```python
from build123d import *

# Parameters (mm, degrees)
F1_DEPTH = 6.35
F2_D     = 4.7625
F3_D     = 3.571875
F4_R     = 5.08


with BuildPart() as f1:
    # F0 (on Front) → F1 (new body)
    with BuildSketch(Plane.XZ):
        Polygon((62.865, 15.748), (12.065, 25.908), (-12.065, 25.908), (-62.865, 15.748), (-62.865, -15.748), (-12.065, -25.908), (12.065, -25.908), (62.865, -15.748), align=None)
    extrude(amount=F1_DEPTH)

    # F2 (through all)
    with Locations(Plane(origin=(0, 0, 0), x_dir=(1, 0, 0), z_dir=(0, 1, 0))):
        with Locations((-13.335, -15.748), (13.335, -15.748), (13.335, 15.748), (-13.335, 15.748)):
            Hole(F2_D / 2)

    # F3 (through all)
    with Locations(Plane(origin=(0, 0, 0), x_dir=(1, 0, 0), z_dir=(0, 1, 0))):
        with Locations((26.035, -9.144), (50.165, -9.144), (50.165, 9.144), (26.035, 9.144), (-26.035, 9.144), (-26.035, -9.144), (-50.165, -9.144), (-50.165, 9.144)):
            Hole(F3_D / 2)

    # F4
    f4_edges = [f1.edges().sort_by_distance(p)[0] for p in [
        (-62.865, -3.175, 15.748),
        (62.865, -3.175, -15.748),
        (-62.865, -3.175, -15.748),
        (62.865, -3.175, 15.748),
        (12.065, -3.175, -25.908),
        (12.065, -3.175, 25.908),
        (-12.065, -3.175, -25.908),
        (-12.065, -3.175, 25.908),
    ]]
    fillet(f4_edges, radius=F4_R)


solid = f1.part
```
Input: part model. Units: mm. Frame: model coordinates. Coordinates: 2 decimals unless noted, no trailing zeros. Loops run counter-clockwise (first coordinate to the right, second up) from the corner with the lowest first, then second, coordinate; pieces in that order, holes last. Notation, with made-up numbers: (78.5, -9.75) -> (91.5, -9.75) arc R17 cw to (91.5, 18.25) -> close; hole circle Ø5 at (-40, 78). An arc over 180 degrees is marked (long way). Use a Markdown table: item, result.
1) Pull-direction query (X, two-part tool) for faces 1 (the cylindrical face through (-27, -3.22, 7.64)), 2 (the flat face through (35.35, -3.13, -21.25)), 3 (the flat face through (-1, -6.35, 0)); classes: released by +X, released by -X, zero draft, split by the parting line, or undercut.
Results found:
| item | result |
|---|---|
| face 1 | undercut |
| face 2 | released by +X |
| face 3 | zero draft |
2) Contact query for flat-ended pins moving along their axis: pin 1 (3 mm diameter, centred on x = -48, y = -4.5, fed in from -Z); pin 2 (3 mm diameter, centred on x = 50.165, z = -9.144, fed in from +Y); pin 3 (2 mm diameter, centred on x = 39, y = -5, fed in from -Z). Output: stop coordinate, or through.
Results found:
| item | result |
|---|---|
| pin 1 | stops at z = -19.02 |
| pin 2 | passes through |
| pin 3 | stops at z = -20.72 |
3) Cut plane A-A (y = -4). Give the number of separate pieces and of enclosed holes in the cut face, then the cut area to 3 significant figures.
Results found:
| item | result |
|---|---|
| separate pieces | 1 |
| enclosed holes | 12 |
| area | 5,320 mm2 |
4) Cut plane C-C (z = 22.5). Return the cut outline in (x, y) (3 decimals), then the cut area to 3 significant figures.
Results found:
| item | result |
|---|---|
| outline | (-29.105, -6.35) -> (29.105, -6.35) -> (29.105, 0) -> (-29.105, 0) -> close |
| area | 370 mm2 |
5) Material intervals for line 1 along X through (y, z) = (-1.25, 14); line 2 along Z through (x, y) = (50.5, -1); line 3 along X through (y, z) = (-1, -8.5) (3 decimals), sorted ascending. Write a range as from..to.
Results found:
| item | result |
|---|---|
| line 1 | x = -62.25..-14.95, -11.72..11.72, 14.95..62.25 |
| line 2 | z = -18.22..-10.9, -7.39..7.39, 10.9..18.22 |
| line 3 | x = -62.865..-51.831, -48.499..-27.701, -24.369..24.369, 27.701..48.499, 51.831..62.865 |
6) Cut plane B-B (x = 55). Return the cut outline in (y, z).
Results found:
| item | result |
|---|---|
| outline | (-6.35, -17.32) -> (0, -17.32) -> (0, 17.32) -> (-6.35, 17.32) -> close |
